Design review of the part shown in the three views and the two pictorial views. Dimensions are in mm from the part's minimum x, y and z. A direction names the side the tool comes from. Coordinates: 2 decimals unless noted, no trailing zeros. Loops run counter-clockwise (first coordinate to the right, second up) from the corner with the lowest first, then second, coordinate; pieces in that order, holes last. Notation, with made-up numbers: M 88,87 L 125,87 A20 cw 125,104 Z; hole C 74,71 d5. An arc over 180 degrees is marked long. Use CSV: the item, a comma, the result in double quotes. Start each with the question number.
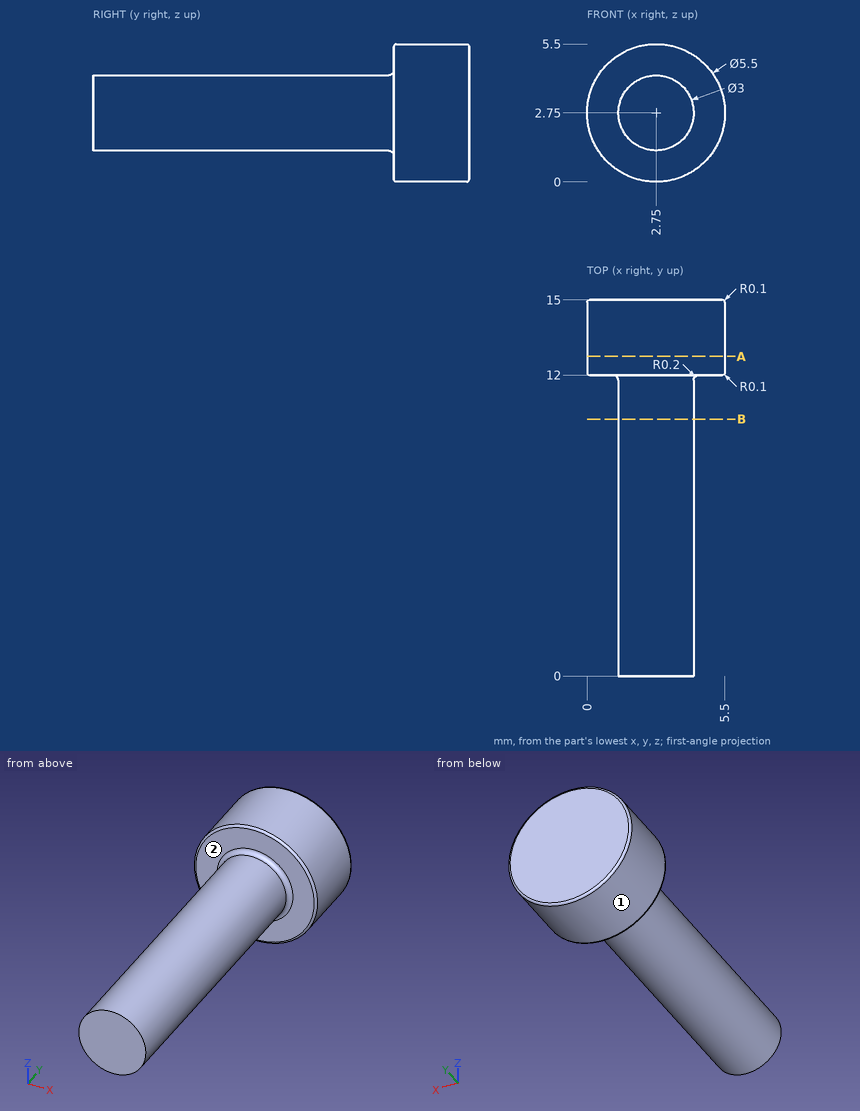
1. For the marked faces 1 and 2, list the 3-axis set-ups (+Z, -Z, +X, -X, +Y, -Y) from which the entire face can be reached by the end or side of a thin tool; tool diameter is ignored.
2. Add section A-A (y = 12.75). Write out the cut boundary in (x, z).
3. Add section B-B (y = 10.25). Write out the cut boundary in (x, z).
4. Insertion check: pin 1 Ø1.5 at (x, y) = (2, 7) entering from -Z. The pin has a flat end and moves straight along its axis. Give the tip position at first contact, or say it passes through.
5. To check wall thickness, follow line 1 along X through (y, z) = (2.25, 2.75); line 2 along Y through (x, z) = (1.05, 1.6); line 3 along X through (y, z) = (13.75, 2.85). State the ranges of each line that lie inside material, in increasing order.
Solved:
1,face 1,"+Y, -Y"
1,face 2,"-Y"
2,outline,"C 2.75,2.75 d5.5"
3,outline,"C 2.75,2.75 d3"
4,pin 1,"stops at z = 1.25"
5,line 1,"x = 1.25 to 4.25"
5,line 2,"y = 12 to 15"
5,line 3,"x = 0 to 5.5"
